```python
from build123d import *

# Parameters (mm, degrees)
EXTRUDE_1_DEPTH          = 7
SKETCH_2_R               = 1.125
CUT_EXTRUDE_2_DEPTH      = 1
CUT_EXTRUDE_2_DEPTH_BACK = 8
SKETCH_4_R               = 1.4
CUT_EXTRUDE_3_DEPTH      = 72
SKETCH_5_R               = 1.4
CUT_EXTRUDE_4_DEPTH      = 8.0000001


with BuildPart() as part:
    # 스케치1 → 보스-돌출1 (new body)
    with BuildSketch(Plane(origin=(0, 0, 0), x_dir=(1, 0, 0), z_dir=(0, 1, 0))):
        with BuildLine():
            Line((0, 21), (45, 21))
            Line((45, 21), (45, 39))
            Line((45, 39), (-26, 39))
            Line((-26, 39), (-26, 0))
            ThreePointArc((-26, 0), (-18.384776311, -18.384776311), (0, -26))
            Line((0, -26), (45, -26))
            Line((45, -26), (45, -21))
            Line((45, -21), (0, -21))
            ThreePointArc((0, -21), (-21, 0), (0, 21))
        make_face()
    extrude(amount=EXTRUDE_1_DEPTH)

    # 스케치2 → 컷-돌출2 (cut, two sides)
    with BuildSketch(Plane(origin=(0, 7, 0), x_dir=(1, 0, 0), z_dir=(0, 1, 0))) as cut_extrude_2_sk:
        with Locations((39.4457939, 35)):
            Circle(SKETCH_2_R)
        with Locations((39.4457939, -23.5)):
            Circle(SKETCH_2_R)
    extrude(amount=CUT_EXTRUDE_2_DEPTH, mode=Mode.SUBTRACT)
    extrude(cut_extrude_2_sk.sketch, amount=-CUT_EXTRUDE_2_DEPTH_BACK, mode=Mode.SUBTRACT)

    # 스케치4 → 컷-돌출3 (cut, through all)
    with BuildSketch(Plane.ZY.offset(26)):
        with Locations((1.986219712, 3.5)):
            Circle(SKETCH_4_R)
    extrude(amount=-CUT_EXTRUDE_3_DEPTH, mode=Mode.SUBTRACT)

    # 스케치5 → 컷-돌출4 (cut, through all)
    with BuildSketch(Plane(origin=(0, 7, 0), x_dir=(1, 0, 0), z_dir=(0, 1, 0))):
        with Locations((16.25, 34)):
            Circle(SKETCH_5_R)
        with Locations((-16.25, 34)):
            Circle(SKETCH_5_R)
    extrude(amount=-CUT_EXTRUDE_4_DEPTH, mode=Mode.SUBTRACT)


solid = part.part
```
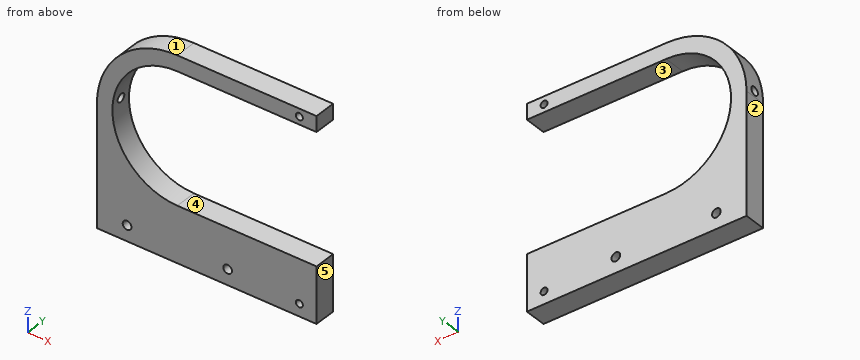
Model file for the job. Use its own axes, mm. Face numbers are marked on the shaded views. A direction names the side the tool comes from. Give positions to 0.01 mm unless a question says otherwise; leave off trailing zeros. Write each loop counter-clockwise with the first axis right and the second up, starting at its lowest first coordinate (ties: lowest second). Pieces come first, ordered by that corner, then holes. Notation, with made-up numbers: (17, -13.5) - (50, -13.5) arc R12 cw to (50, 9.5) - close; hole circle Ø4 at (80, -10.5). An arc over 180 degrees is marked (long way). One line per question, with ' | ' between items. Start each with the question number.
(1) 3-axis set-ups, long thin cutter, end or side, ignore diameter. For the marked faces 4 and 5: which of +Z, -Z, +X, -X, +Y, -Y reach the whole face in a straight line?
(2) Slice it at C-C on x = 2. Write the cut outline in (y, z).
(3) Slice it at A-A on z = 23.5. Write the cut outline in (x, y), plus the area to 3 significant figures.
(4) Wall check: line 1 along Z through (x, y) = (16.25, 2); line 2 along Z through (x, y) = (39, 5); line 3 along X through (y, z) = (4.25, -34). Give the ranges that are in metal, low to high. Write a range as from..to.
(5) Slice it at B-B on y = 3.5. Write the cut outline in (x, z) (3 decimals).
(6) Two-plate mould, pull along Z, no slides. Class the marked faces 1, 2 and 3: +Z half, -Z half, draft (parallel to the pull), parting line (faces both ways), or undercut.
(7) Pin check, flat tip, straight feed: P1, Ø4.5, axis at x = 16.25, z = -34, coming from the -Y side. Stop position of the tip, or through.
(8) Slice it at D-D on z = -12. Write the cut outline in (x, y), plus the area to 3 significant figures.
Results below:
1) face 4: +X, +Y, -Y | face 5: +Z, -Z, +X, +Y, -Y
2) outline: (0, -39) - (7, -39) - (7, -21) - (0, -21) - close; (0, 21) - (7, 21) - (7, 26) - (0, 26) - close
3) outline: (-11.12, 0) - (38.32, 0) - (38.32, 7) - (-11.12, 7) - close; (40.57, 0) - (45, 0) - (45, 7) - (40.57, 7) - close | area: 377 mm^2
4) line 1: -39..-35.4, -32.6..-21, 21..26 | line 2: -39..-36.03, -33.97..-21, 21..22.47, 24.53..26 | line 3: -26..-17.65, -14.85..14.85, 17.65..38.93, 39.96..45
5) outline: (-26, -39) - (45, -39) - (45, -21) - (0, -21) arc R21 cw to (-20.992, 0.586) - (-25.993, 0.586) arc R26 ccw to (-26, 0) - close; (-25.779, 3.386) - (-20.725, 3.386) arc R21 cw to (0, 21) - (45, 21) - (45, 26) - (0, 26) arc R26 ccw to start; hole circle Ø2.8 at (-16.25, -34); hole circle Ø2.8 at (16.25, -34); hole circle Ø2.25 at (39.446, -35); hole circle Ø2.25 at (39.446, 23.5)
6) face 1: +Z half | face 2: draft | face 3: undercut
7) P1: y = 0
8) outline: (-26, 0) - (-17.23, 0) - (-17.23, 7) - (-26, 7) - close | area: 61.4 mm^2
